from build123d import *

# Parameters (mm, degrees)
SKETCH1_W            = 5
SKETCH1_H            = 54
BOSS_EXTRUDE1_DEPTH  = 4
SKETCH3_W            = 16
SKETCH3_H            = 16
BOSS_EXTRUDE2_DEPTH  = 4
SKETCH6_W            = 5
SKETCH6_H            = 4
BOSS_EXTRUDE5_DEPTH  = 5
SKETCH10_W           = 30
SKETCH10_H           = 20
BOSS_EXTRUDE9_DEPTH  = 6
CUT_EXTRUDE2_REACH   = 54.903
SKETCH7_R            = 2
CUT_EXTRUDE3_REACH   = 54.903
SKETCH4_R            = 5
SKETCH12_W           = 16
SKETCH12_H           = 16
CUT_EXTRUDE4_DEPTH   = 2
CUT_EXTRUDE5_DEPTH   = 4
CUT_EXTRUDE6_REACH   = 78.804
SKETCH14_R           = 5
FILLET1_R            = 5
FILLET1_OF_MIRROR2_R = 5
CUT_EXTRUDE7_REACH   = 54.903
FILLET2_R            = 2.5


with BuildPart() as part:
    # Sketch1 → Boss-Extrude1 (new body)
    with BuildSketch(Plane(origin=(0, 0, 0), x_dir=(1, 0, 0), z_dir=(0, 1, 0))):
        with Locations((-2.5, 0)):
            Rectangle(SKETCH1_W, SKETCH1_H)
    extrude(amount=BOSS_EXTRUDE1_DEPTH)

    # Sketch3 → Boss-Extrude2 (add)
    with BuildSketch(Plane(origin=(0, 0, 0), x_dir=(1, 0, 0), z_dir=(0, 1, 0))):
        with Locations((8, 0)):
            Rectangle(SKETCH3_W, SKETCH3_H)
    extrude(amount=BOSS_EXTRUDE2_DEPTH)

    # Sketch6 → Boss-Extrude5 (add, along a direction that is not the sketch's normal)
    with BuildSketch(Plane.XY.offset(27)):
        with Locations((-2.5, 2)):
            Rectangle(SKETCH6_W, SKETCH6_H)
    boss_extrude5 = extrude(amount=BOSS_EXTRUDE5_DEPTH, dir=(0, -0.5827823156195225, 0.8126283114691164))

    # Mirror1: Boss-Extrude5 across plane
    add(boss_extrude5.mirror(Plane.XY))

    # Sketch10 → Boss-Extrude9 (add)
    with BuildSketch(Plane.XY.offset(31.063141557)):
        with Locations((-15, -8.913911578)):
            Rectangle(SKETCH10_W, SKETCH10_H)
    boss_extrude9 = extrude(amount=BOSS_EXTRUDE9_DEPTH)

    # Sketch7 → Cut-Extrude2 (cut, up to next)
    with BuildSketch(Plane(origin=(0, 4, 0), x_dir=(1, 0, 0), z_dir=(0, 1, 0)), mode=Mode.PRIVATE) as cut_extrude2_sk1:
        with Locations(Location((-2.5, 0, 0), (0, 0, 270))):
            Circle(SKETCH7_R)
    cut_extrude2_tool1 = extrude(cut_extrude2_sk1.sketch, amount=-CUT_EXTRUDE2_REACH, mode=Mode.PRIVATE) & part.part
    # Sketch7 → Cut-Extrude2 (cut, up to next)
    with BuildSketch(Plane(origin=(0, 4, 0), x_dir=(1, 0, 0), z_dir=(0, 1, 0)), mode=Mode.PRIVATE) as cut_extrude2_sk2:
        with Locations(Location((-2.5, 15, 0), (0, 0, 270))):
            Circle(SKETCH7_R)
    cut_extrude2_tool2 = extrude(cut_extrude2_sk2.sketch, amount=-CUT_EXTRUDE2_REACH, mode=Mode.PRIVATE) & part.part
    # Sketch7 → Cut-Extrude2 (cut, up to next)
    with BuildSketch(Plane(origin=(0, 4, 0), x_dir=(1, 0, 0), z_dir=(0, 1, 0)), mode=Mode.PRIVATE) as cut_extrude2_sk3:
        with Locations(Location((-2.5, -15, 0), (0, 0, 270))):
            Circle(SKETCH7_R)
    cut_extrude2_tool3 = extrude(cut_extrude2_sk3.sketch, amount=-CUT_EXTRUDE2_REACH, mode=Mode.PRIVATE) & part.part
    add(cut_extrude2_tool1.solids().sort_by_distance((-2.5, 4, 0))[0], mode=Mode.SUBTRACT)
    add(cut_extrude2_tool2.solids().sort_by_distance((-2.5, 4, -15))[0], mode=Mode.SUBTRACT)
    add(cut_extrude2_tool3.solids().sort_by_distance((-2.5, 4, 15))[0], mode=Mode.SUBTRACT)

    # Sketch4 → Cut-Extrude3 (cut, up to next)
    with BuildSketch(Plane(origin=(0, 4, 0), x_dir=(1, 0, 0), z_dir=(0, 1, 0)), mode=Mode.PRIVATE) as cut_extrude3_sk1:
        with Locations(Location((8, 0, 0), (0, 0, 270))):
            Circle(SKETCH4_R)
    cut_extrude3_tool1 = extrude(cut_extrude3_sk1.sketch, amount=-CUT_EXTRUDE3_REACH, mode=Mode.PRIVATE) & part.part
    add(cut_extrude3_tool1.solids().sort_by_distance((8, 4, 0))[0], mode=Mode.SUBTRACT)

    # Sketch12 → Cut-Extrude4 (cut)
    with BuildSketch(Plane.XZ):
        with Locations((8, 0)):
            Rectangle(SKETCH12_W, SKETCH12_H)
    extrude(amount=-CUT_EXTRUDE4_DEPTH, mode=Mode.SUBTRACT)

    # Sketch13 → Cut-Extrude5 (cut)
    with BuildSketch(Plane(origin=(0, 0, 31.063141557), x_dir=(-1, 0, 0), z_dir=(0, 0, -1))):
        Polygon((30, 1.086088422), (5, 1.086088422), (5, -2.913911578), (0, -2.913911578), (0, -18.913911578), (30, -18.913911578), align=None)
    cut_extrude5 = extrude(amount=-CUT_EXTRUDE5_DEPTH, mode=Mode.SUBTRACT)

    # Sketch14 → Cut-Extrude6 (cut, up to next)
    with BuildSketch(Plane.XY.offset(37.063141557), mode=Mode.PRIVATE) as cut_extrude6_sk1:
        with Locations((-22, -11.413911578)):
            Circle(SKETCH14_R)
    cut_extrude6_tool1 = extrude(cut_extrude6_sk1.sketch, amount=-CUT_EXTRUDE6_REACH, mode=Mode.PRIVATE) & part.part
    cut_extrude6 = cut_extrude6_tool1.solids().sort_by_distance((-22, -11.413912, 37.063142))[0]
    add(cut_extrude6, mode=Mode.SUBTRACT)

    # Fillet1
    fillet1_edges = [part.edges().sort_by_distance(p)[0] for p in [
        (0, -18.913911578, 36.063141557),
        (-30, 1.086088422, 36.063141557),
        (-30, -18.913911578, 36.063141557),
    ]]
    fillet(fillet1_edges, radius=FILLET1_R)

    # Mirror2: Boss-Extrude9, Cut-Extrude5, Cut-Extrude6 across plane
    add(boss_extrude9.mirror(Plane.XY))
    add(cut_extrude5.mirror(Plane.XY), mode=Mode.SUBTRACT)
    add(cut_extrude6.mirror(Plane.XY), mode=Mode.SUBTRACT)

    # Fillet1 of Mirror2
    fillet1_of_mirror2_edges = [part.edges().sort_by_distance(p)[0] for p in [
        (0, -18.913911578, -36.063141557),
        (-30, 1.086088422, -36.063141557),
        (-30, -18.913911578, -36.063141557),
    ]]
    fillet(fillet1_of_mirror2_edges, radius=FILLET1_OF_MIRROR2_R)

    # Sketch15 → Cut-Extrude7 (cut, up to next)
    with BuildSketch(Plane(origin=(0, 4, 0), x_dir=(1, 0, 0), z_dir=(0, 1, 0)), mode=Mode.PRIVATE) as cut_extrude7_sk1:
        with BuildLine():
            Line((8, 5), (8, 8))
            Line((8, 8), (16, 8))
            Line((16, 8), (16, -8))
            Line((16, -8), (8, -8))
            Line((8, -8), (8, -5))
            ThreePointArc((8, -5), (13, 0), (8, 5))
        make_face()
    cut_extrude7_tool1 = extrude(cut_extrude7_sk1.sketch, amount=-CUT_EXTRUDE7_REACH, mode=Mode.PRIVATE) & part.part
    add(cut_extrude7_tool1.solids().sort_by_distance((8.178885, 4, -6.5))[0], mode=Mode.SUBTRACT)

    # Fillet2
    fillet2_edges = [part.edges().sort_by_distance(p)[0] for p in [
        (8, 3, 8),
        (8, 3, -8),
    ]]
    fillet(fillet2_edges, radius=FILLET2_R)


solid = part.part
Geometry check sheet. Reference: the model listing, model coordinates, mm. A direction names the side the tool comes from. Round coordinates to 2 decimals unless told otherwise and drop trailing zeros. Order: outer loops, then holes, each group sorted by start corner. A loop starts at its lowest first (then second) coordinate and runs counter-clockwise, first axis right, second up. Notation, with made-up numbers: M 35.25,-2 L 70.25,-2 A29 cw 70.25,37 Z; hole C 57.5,86 d3. An arc over 180 degrees is marked long. Answer in a Markdown table with one row per item. Add a question column.
Item 1: Sectioned sample at C-C, the plane y = -5.25. Enter the section's corners in (x, z).
Item 2: Set-up check for faces 1 (the face through (-3, -2.914, -33)), 2 (the face through (-28.574, -0.417, 36.077)), 3 (the face through (-15, -9, 35.063)), 4 (the face through (-9.9, 1.086, -35.4)): record each of +Z, -Z, +X, -X, +Y, -Y from which the full face is reachable in a straight line by a thin tool's end or side.
Item 3: Sectioned sample at D-D, the plane y = -10.25. Enter the section's corners in (x, z), plus the area to 3 significant figures.
Item 4: Material ranges on L1, parallel to Z at x = -18.5, y = -3.5; L2, parallel to X at y = 2.85, z = -15; L3, parallel to X at y = 2.9, z = 0, recorded low to high. Write a range as [from, to].
Item 5: Draft check along Z on faces 5 (the face through (-5, 1, 0)), 6 (the face through (-15, -9, -37.063)), 7 (the face through (-26.995, -11.194, 36.077)). Enter one of: released by +Z, released by -Z, zero draft, split by the parting line, or undercut.
Item 6: Depth check by flat-ended pin: pin 1 Ø1 at (x, z) = (-3.5, -1) entering from +Y; pin 2 Ø3 at (x, z) = (-3, -32.5) entering from -Y; pin 3 Ø3.5 at (y, z) = (0.5, 4) entering from -X; pin 4 Ø1.6 at (x, y) = (3, 3) entering from -Z. Enter the tip coordinate at first touch or a pass-through.
Item 7: Sectioned sample at B-B, the plane z = 15. Enter the section's corners in (x, y).
Item 8: Sectioned sample at A-A, the plane x = -22. Enter the section's corners in (y, z).
Filled in:
| question | item | result |
|---|---|---|
| 1 | outline | M -30,-37.06 L 0,-37.06 L 0,-35.06 L -30,-35.06 Z; M -30,35.06 L 0,35.06 L 0,37.06 L -30,37.06 Z |
| 2 | face 1 | +X, -X, -Y |
| 2 | face 2 | +Z, -Z, -X, +Y |
| 2 | face 3 | -X, -Y |
| 2 | face 4 | -Z, +X, -X, +Y |
| 3 | outline | M -30,-37.06 L -26.86,-37.06 L -26.86,-35.06 L -30,-35.06 Z; M -30,35.06 L -26.86,35.06 L -26.86,37.06 L -30,37.06 Z; M -17.14,-37.06 L 0,-37.06 L 0,-35.06 L -17.14,-35.06 Z; M -17.14,35.06 L 0,35.06 L 0,37.06 L -17.14,37.06 Z |
| 3 | area | 81.1 mm² |
| 4 | L1 | z = [-37.06, -35.06], [35.06, 37.06] |
| 4 | L2 | x = [-5, -4.5], [-0.5, 0] |
| 4 | L3 | x = [-5, -4.5], [-0.5, 3] |
| 5 | face 5 | undercut |
| 5 | face 6 | released by -Z |
| 5 | face 7 | zero draft |
| 6 | pin 1 | passes through |
| 6 | pin 2 | stops at y = -2.91 |
| 6 | pin 3 | stops at x = -5 |
| 6 | pin 4 | stops at z = -8 |
| 7 | outline | M -5,0 L -4.5,0 L -4.5,4 L -5,4 Z; M -0.5,0 L 0,0 L 0,4 L -0.5,4 Z |
| 8 | outline | M -18.91,-37.06 L -16.41,-37.06 L -16.41,-35.06 L -18.91,-35.06 Z; M -18.91,35.06 L -16.41,35.06 L -16.41,37.06 L -18.91,37.06 Z; M -6.41,-37.06 L 1.09,-37.06 L 1.09,-35.06 L -6.41,-35.06 Z; M -6.41,35.06 L 1.09,35.06 L 1.09,37.06 L -6.41,37.06 Z |
